```python
from build123d import *

# Parameters (mm, degrees)
FILLET_1_R         = 5
SKETCH_3_W         = 15
SKETCH_3_H         = 5
EXTRUDE_1_DEPTH    = 35
M4X0_7_1_D         = 3.3
M4X0_7_1_DEPTH     = 11.5
M4X0_7_1_TIP       = 0.991420021
SKETCH_6_W         = 0.5
SKETCH_6_H         = 1
CUT_EXTRUDE1_DEPTH = 1.8


with BuildPart() as part:
    # 스케치1 → 회전1 (revolve)
    with BuildSketch(Plane.XY, mode=Mode.PRIVATE) as revolve_1_sk:
        Polygon((0, 82.5), (4, 82.5), (4, 61), (31.5, 61), (31.5, 0), (0, 0), align=None)
    revolve(revolve_1_sk.sketch.rotate(Axis((0, 0, 0), (0, 1, 0)), 90), axis=Axis((0, 0, 0), (0, 1, 0)))

    # 필렛1
    fillet_1_edges = [part.edges().sort_by_distance(p)[0] for p in [
        (0, 0, 31.5),
        (0, 61, 31.5),
    ]]
    fillet(fillet_1_edges, radius=FILLET_1_R)

    # 스케치3 → 보스-돌출1 (add)
    with BuildSketch(Plane(origin=(0, 0, 0), x_dir=(0, 0, -1), z_dir=(1, 0, 0))):
        with Locations((0, 58.5)):
            Rectangle(SKETCH_3_W, SKETCH_3_H)
    extrude(amount=EXTRUDE_1_DEPTH)

    # M4x0.7 나사 구멍1
    with Locations(Plane(origin=(0, 61, 0), x_dir=(1, 0, 0), z_dir=(0, 1, 0))):
        with Locations((10.606601718, 10.606601718), (15.556349186, 15.556349186), (10.606601718, -10.606601718), (15.556349186, -15.556349186), (-10.606601718, -10.606601718), (-15.556349186, -15.556349186), (-10.606601718, 10.606601718), (-15.556349186, 15.556349186)):
            Hole(M4X0_7_1_D / 2, depth=M4X0_7_1_DEPTH)
            with Locations((0, 0, -(M4X0_7_1_DEPTH + M4X0_7_1_TIP / 2))):  # 118° drill point
                Cone(0, M4X0_7_1_D / 2, M4X0_7_1_TIP, mode=Mode.SUBTRACT)

    # 스케치6 → 컷-회전1 (revolve, cut)
    with BuildSketch(Plane(origin=(0, 0, 0), x_dir=(0, 0, -1), z_dir=(1, 0, 0))):
        with Locations((3.75, 81)):
            Rectangle(SKETCH_6_W, SKETCH_6_H)
    revolve(axis=Axis((0, 82.5, 0), (0, -1, 0)), mode=Mode.SUBTRACT)

    # Sketch3 → Cut-Extrude1 (cut)
    with BuildSketch(Plane(origin=(2.845698698, 82.5, 4), x_dir=(0, 1, 0), z_dir=(0, 0, -1))):
        with BuildLine():
            Line((-2.5, -1.345698698), (-20.5, -1.345698698))
            ThreePointArc((-20.5, -1.345698698), (-22, -2.845698698), (-20.5, -4.345698698))
            Line((-20.5, -4.345698698), (-2.5, -4.345698698))
            ThreePointArc((-2.5, -4.345698698), (-1, -2.845698698), (-2.5, -1.345698698))
        make_face()
    extrude(amount=CUT_EXTRUDE1_DEPTH, mode=Mode.SUBTRACT)


solid = part.part
```
Geometry: final body of the model. Coordinates: model frame, mm. A direction names the side the tool comes from. Give positions to 0.01 mm unless a question says otherwise; leave off trailing zeros. Order: outer loops, then holes, each group sorted by start corner. A loop starts at its lowest first (then second) coordinate and runs counter-clockwise, first axis right, second up. Notation, with made-up numbers: M 11,85 L 46,85 A23 ccw 46,104 Z; hole C -26,18.5 d8. An arc over 180 degrees is marked long. Answer as CSV lines item,"result". Start each with the question number.
1) First-contact query: P1, Ø12, axis at y = 38.5, z = -13.5, coming from the -X side; P2, Ø12, axis at y = 51, z = 16, coming from the +X side; P3, Ø0.5, axis at y = 69, z = 3, coming from the -X side; P4, Ø6, axis at x = 8, y = 71.5, coming from the +Z side. Flat tips, straight axial feed; report the tip coordinate or a pass-through.
2) Cut plane A-A (z = 0). Output: boundary loops of the cut face in (x, y).
3) Cut plane C-C (y = 44.5). Output: boundary loops of the cut face in (x, z).
4) Set-up query: faces 1 (the cylindrical face through (17.205, 55.17, -15.629)), 2 (the flat face through (0, 0, 0)). Return all of +Z, -Z, +X, -X, +Y, -Y with unobstructed straight access to the full face (end or side cutting, diameter ignored); none if empty.
5) Cut plane B-B (y = 74). Output: boundary loops of the cut face in (x, z), then the cut area to 3 significant figures.
6) Line query: line 1 (Y direction, x = -12, z = -9); line 2 (Z direction, x = 9.5, y = 57); line 3 (Z direction, x = -23, y = 43). Output: solid intervals per line, ascending. Write a range as from..to.
7) Mould query, pull axis Z, two halves, no side actions, for faces 3 (the conical face through (-15.59, 48.68, -15.84)), 4 (the flat face through (4, 61, -6)), 5 (the flat face through (32, 59, -7.5)). Classes: +Z half, -Z half, draft (parallel to the pull), parting line (faces both ways), or undercut.
Findings below:
1,P1,"stops at x = -30.59"
1,P2,"stops at x = 29.87"
1,P3,"stops at x = -2.9"
1,P4,"passes through"
2,outline,"M -31.5,5 A5 ccw -26.5,0 L 26.5,0 A5 ccw 31.5,5 L 31.5,56 L 35,56 L 35,61 L 4,61 L 4,80.5 L 3.5,80.5 L 3.5,81.5 L 4,81.5 L 4,82.5 L -4,82.5 L -4,81.5 L -3.5,81.5 L -3.5,80.5 L -4,80.5 L -4,61 L -26.5,61 A5 ccw -31.5,56 Z"
3,outline,"C 0,0 d63"
4,face 1,"+Y"
4,face 2,"+Z, -Z, +X, -X, -Y"
5,outline,"M -1.5,2.2 L -1.5,3.71 A4 ccw long 1.5,3.71 L 1.5,2.2 Z"
5,area,"45.2 mm²"
6,line 1,"y = 0..61"
6,line 2,"z = -29.93..-11.83, -9.38..9.38, 11.83..29.93"
6,line 3,"z = -21.52..21.52"
7,face 3,"undercut"
7,face 4,"draft"
7,face 5,"-Z half"
